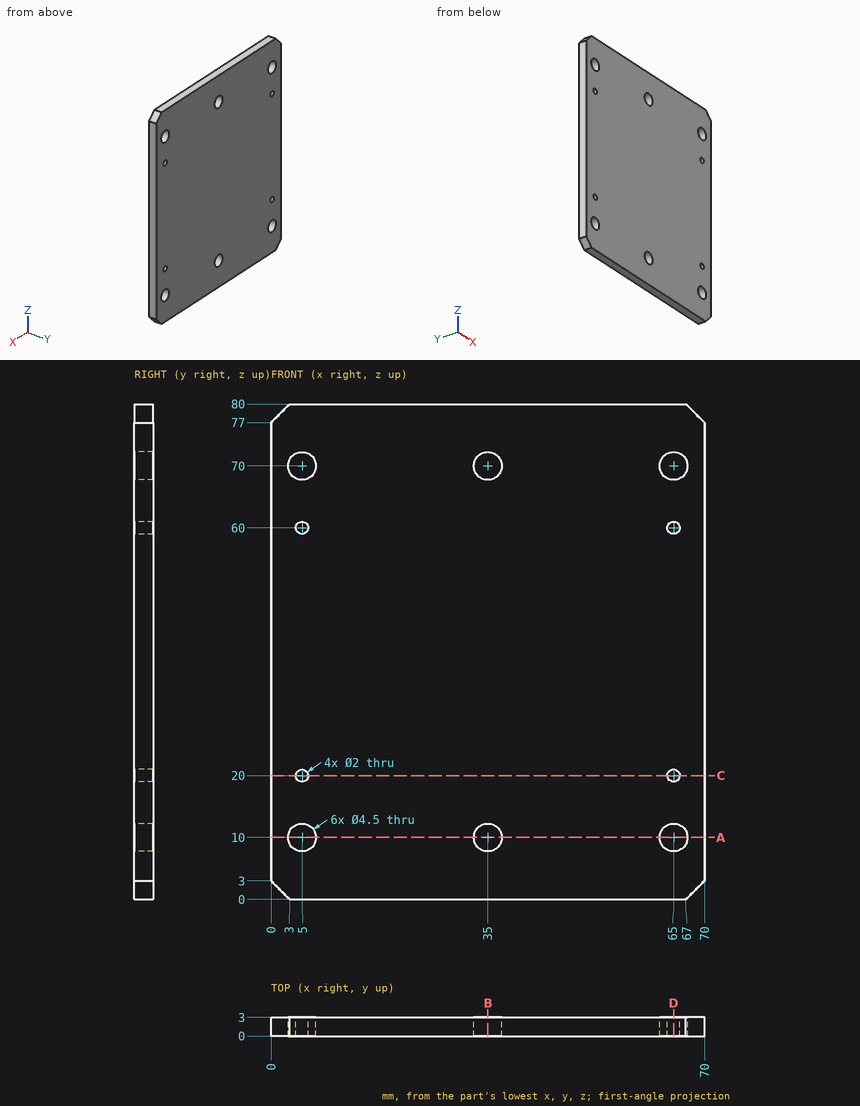
Input: dimensioned drawing with shaded views. Units: mm. Origin: part minimum x, y, z. Coordinates: 2 decimals unless noted, no trailing zeros. Loops run counter-clockwise (first coordinate to the right, second up) from the corner with the lowest first, then second, coordinate; pieces in that order, holes last. Notation, with made-up numbers: M 17,60 L 42,60 A10 cw 42,70 Z; hole C 61,-4 d3. An arc over 180 degrees is marked long. One line per item, written item: value. Start each with the question number.
1) Cut plane A-A (z = 10). Return loops of the section in (x, y).
2) Cut plane B-B (x = 35). Return loops of the section in (y, z), then the cut area to 3 significant figures.
3) Cut plane C-C (z = 20). Return loops of the section in (x, y), then the cut area to 3 significant figures.
4) Cut plane D-D (x = 65). Return loops of the section in (y, z), then the cut area to 3 significant figures.
5) Pin query (flat end, axial travel): P1, Ø4, axis at x = 35, z = 70, coming from the -Y side. Return the tip coordinate at first contact, or that it passes through.
6) Material intervals for L1, parallel to X at y = 1.1, z = 60; L2, parallel to X at y = 2.3, z = 10; L3, parallel to Z at x = 67, y = 1.7, sorted ascending. Write a range as from..to.
Evaluation:
1. outline: M 0,0 L 2.75,0 L 2.75,3 L 0,3 Z; M 7.25,0 L 32.75,0 L 32.75,3 L 7.25,3 Z; M 37.25,0 L 62.75,0 L 62.75,3 L 37.25,3 Z; M 67.25,0 L 70,0 L 70,3 L 67.25,3 Z
2. outline: M 0,0 L 3,0 L 3,7.75 L 0,7.75 Z; M 0,12.25 L 3,12.25 L 3,67.75 L 0,67.75 Z; M 0,72.25 L 3,72.25 L 3,80 L 0,80 Z
2. area: 213 mm^2
3. outline: M 0,0 L 4,0 L 4,3 L 0,3 Z; M 6,0 L 64,0 L 64,3 L 6,3 Z; M 66,0 L 70,0 L 70,3 L 66,3 Z
3. area: 198 mm^2
4. outline: M 0,0 L 3,0 L 3,7.75 L 0,7.75 Z; M 0,12.25 L 3,12.25 L 3,19 L 0,19 Z; M 0,21 L 3,21 L 3,59 L 0,59 Z; M 0,61 L 3,61 L 3,67.75 L 0,67.75 Z; M 0,72.25 L 3,72.25 L 3,80 L 0,80 Z
4. area: 201 mm^2
5. P1: through
6. L1: 0..4, 6..64, 66..70
6. L2: 0..2.75, 7.25..32.75, 37.25..62.75, 67.25..70
6. L3: 0..8.97, 11.03..68.97, 71.03..80
